Model file for the job. Use its own axes, mm. Coordinates: 2 decimals unless noted, no trailing zeros. Order: outer loops, then holes, each group sorted by start corner. A loop starts at its lowest first (then second) coordinate and runs counter-clockwise, first axis right, second up.
Autodesk Inventor part; units mm, degrees
ref_plane "YZ Plane" through (0, 0, 0) normal (1, 0, 0) x (0, 1, 0)
ref_plane "XZ Plane" through (0, 0, 0) normal (0, 1, 0) x (-1, 0, 0)
ref_plane "XY Plane" through (0, 0, 0) normal (0, 0, 1) x (1, 0, 0)
sketch "スケッチ1" plane through (0, 0, 0) normal (0, 0, 1) x (1, 0, 0)
  circle A0 centre (0, 0) radius 87.5
  circle A1 centre (0, 0) radius 100
  circle A2 centre (0, 0) radius 93.75 construction
  circle A3 centre (0, 93.75) radius 4
  circle A4 centre (93.75, 0) radius 4
  circle A5 centre (0, -93.75) radius 4
  circle A6 centre (-93.75, 0) radius 4
  dimension "d0" = 175
  dimension "d1" = 200
  dimension "d2" = 187.5
  dimension "d3" = 8
  dimension "d4" = 8
  dimension "d5" = 8
  dimension "d6" = 8
extrude "押し出し1" add sketch "スケッチ1" along normal blind 8.5
properties part number "ベアリング 外側"
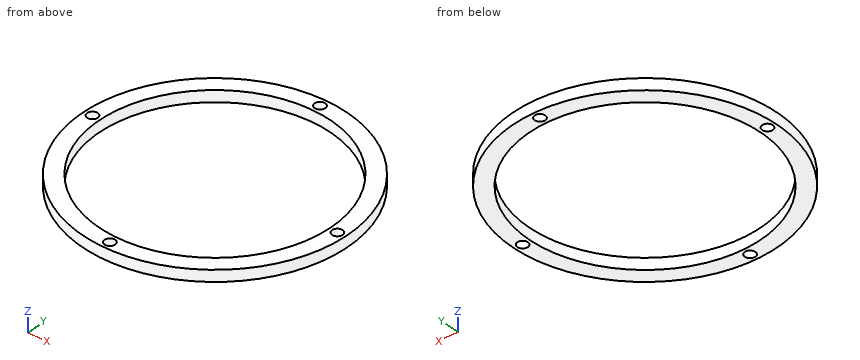
Q1. Cut at B-B, the plane x = 0. List the corners of the cut face in (y, z).
Established:
outline: (-100, 0) - (-97.75, 0) - (-97.75, 8.5) - (-100, 8.5) - close; (-89.75, 0) - (-87.5, 0) - (-87.5, 8.5) - (-89.75, 8.5) - close; (87.5, 0) - (89.75, 0) - (89.75, 8.5) - (87.5, 8.5) - close; (97.75, 0) - (100, 0) - (100, 8.5) - (97.75, 8.5) - close
Q2. Cut at A-A, the plane y = -44. List the corners of the cut face in (x, z), plus the area to 3 significant figures.
Established:
outline: (-89.8, 0) - (-75.63, 0) - (-75.63, 8.5) - (-89.8, 8.5) - close; (75.63, 0) - (89.8, 0) - (89.8, 8.5) - (75.63, 8.5) - close
area: 241 mm2
Q3. Drop flat-ended pins along their axis: P1, Ø5, axis at x = -51, z = 3.5, coming from the -Y side; P2, Ø1, axis at y = 76, z = 2, coming from the -X side; P3, Ø5, axis at x = -55, y = 63, coming from the +Z side; P4, Ø3, axis at y = -56, z = 5, coming from the -X side. Give the stop position or say it passes through.
Established:
P1: stops at y = -87.45
P2: stops at x = -65.57
P3: passes through
P4: stops at x = -83.84
Q4. Cut at C-C, the plane x = 72. List the corners of the cut face in (y, z), plus the area to 3 significant figures.
Established:
outline: (-69.4, 0) - (-49.72, 0) - (-49.72, 8.5) - (-69.4, 8.5) - close; (49.72, 0) - (69.4, 0) - (69.4, 8.5) - (49.72, 8.5) - close
area: 334 mm2
Q5. Probe line 1 (Y direction, x = 0, z = 3.75); line 2 (X direction, y = -54.5, z = 3.75); line 3 (X direction, y = 47.5, z = 2). List the from-to ranges inside material, lowest first.
Established:
line 1: y = -100 to -97.75, -89.75 to -87.5, 87.5 to 89.75, 97.75 to 100
line 2: x = -83.84 to -68.45, 68.45 to 83.84
line 3: x = -88 to -73.48, 73.48 to 88
